```python
from build123d import *

# Parameters (mm, degrees)
F0_W     = 8
F0_H     = 3.175
F0_R     = 1.5
F0_W_2   = 3.175
F0_H_2   = 4
F0_R_2   = 1
F0_W_3   = 24
F0_H_3   = 12.5
F1_DEPTH = 3.175


# Not quite as in the source:
# - a length typed as a fraction of an inch, garbled in the dataset ("3 / 203.2 mm" for 3/8 in), is restored


with BuildPart() as f1:
    # F0 (on Top) → F1 (new body)
    with BuildSketch(Plane.XY):
        Polygon((-34.1063038088, 0.9337500209), (-34.1063038088, -28.6537499791), (9.0686961912, -28.6537499791), (9.0686961912, 0.9337500209), (-7.9313038088, 0.9337500209), (-7.9313038088, 20.1087500209), (-17.1063038088, 20.1087500209), (-17.1063038088, 0.9337500209), align=None)
        with Locations((-23.9313038088, -21.0662499791)):
            Rectangle(F0_W, F0_H, mode=Mode.SUBTRACT)
        with Locations((-29.5188038088, -10.9787499791)):
            Circle(F0_R, mode=Mode.SUBTRACT)
        with Locations((-29.5188038088, -4.4787499791)):
            Rectangle(F0_W_2, F0_H_2, mode=Mode.SUBTRACT)
        with Locations((-23.9313038088, -8.3162499791)):
            Circle(F0_R_2, mode=Mode.SUBTRACT)
        with Locations((-12.4313038088, -21.0662499791)):
            Circle(F0_R, mode=Mode.SUBTRACT)
        with Locations((-0.9313038088, -21.0662499791)):
            Rectangle(F0_W, F0_H, mode=Mode.SUBTRACT)
        with Locations((-9.4313038088, -8.3162499791)):
            Rectangle(F0_W_3, F0_H_3, mode=Mode.SUBTRACT)
        with Locations((5.0686961912, -8.3162499791)):
            Circle(F0_R_2, mode=Mode.SUBTRACT)
        with BuildLine():
            ThreePointArc((-14.1063038088, 15.5212500209), (-12.5188038088, 17.1087500209), (-10.9313038088, 15.5212500209))
            Line((-10.9313038088, 15.5212500209), (-10.9313038088, 2.5212500209))
            ThreePointArc((-10.9313038088, 2.5212500209), (-12.5188038088, 0.9337500209), (-14.1063038088, 2.5212500209))
            Line((-14.1063038088, 2.5212500209), (-14.1063038088, 15.5212500209))
        make_face(mode=Mode.SUBTRACT)
    extrude(amount=F1_DEPTH)


solid = f1.part
```
Geometry check sheet. Reference: the model listing, model coordinates, mm. A direction names the side the tool comes from. Coordinates: 2 decimals unless noted, no trailing zeros. Loops run counter-clockwise (first coordinate to the right, second up) from the corner with the lowest first, then second, coordinate; pieces in that order, holes last. Notation, with made-up numbers: (59, 83.25) - (109, 83.25) arc R15 ccw to (109, 104.25) - close; hole circle Ø2 at (83, 72.5). An arc over 180 degrees is marked (long way). One line per item, written item: value. Start each with the question number.
(1) Cross-section at B-B on y = -13.5. Enter the section's corners in (x, z) (3 decimals).
(2) Cross-section at C-C on x = -2.5. Enter the section's corners in (y, z) (3 decimals), plus the area to 3 significant figures.
(3) Depth check by flat-ended pin: P1, Ø1.6, axis at y = 12, z = 1, coming from the -X side; P2, Ø1.6, axis at y = 8, z = 1.5, coming from the +X side; P3, Ø1, axis at x = -3, z = 1.5, coming from the +Y side. Enter the tip coordinate at first touch or a pass-through.
(4) Cross-section at D-D on y = -20.5. Enter the section's corners in (x, z) (3 decimals), plus the area to 3 significant figures.
(5) Tool access check on faces 4 (the flat face through (-25, 0.934, 2)), 5 (the cylindrical face through (-12.55, 17.11, 1.57)), 6 (the flat face through (9.069, -14, 2)). Record the directions out of +Z, -Z, +X, -X, +Y, -Y that give a thin tool (end or side, any length) a straight path to the whole face; none if there is none.
(6) Mould release check, pull along Y, two halves, no side actions. Record for faces 1 (the flat face through (-13, -15, 3.175)), 2 (the flat face through (-27.931, -21, 2)), 3 (the flat face through (1, 0.934, 2)): released by +Y, released by -Y, zero draft, split by the parting line, or undercut.
(7) Material ranges on line 1 (Y direction, x = -21, z = 1.95); line 2 (Y direction, x = -10, z = 2.7); line 3 (Y direction, x = -26.5, z = 1.3), recorded low to high. Write a range as [from, to].
(8) Cross-section at A-A on x = -26. Enter the section's corners in (y, z) (3 decimals).
Results below:
1. outline: (-34.106, 0) - (-21.431, 0) - (-21.431, 3.175) - (-34.106, 3.175) - close; (2.569, 0) - (9.069, 0) - (9.069, 3.175) - (2.569, 3.175) - close
2. outline: (-28.654, 0) - (-22.654, 0) - (-22.654, 3.175) - (-28.654, 3.175) - close; (-19.479, 0) - (-14.566, 0) - (-14.566, 3.175) - (-19.479, 3.175) - close; (-2.066, 0) - (0.934, 0) - (0.934, 3.175) - (-2.066, 3.175) - close
2. area: 44.2 mm2
3. P1: stops at x = -17.11
3. P2: stops at x = -7.93
3. P3: stops at y = 0.93
4. outline: (-34.106, 0) - (-27.931, 0) - (-27.931, 3.175) - (-34.106, 3.175) - close; (-19.931, 0) - (-13.82, 0) - (-13.82, 3.175) - (-19.931, 3.175) - close; (-11.042, 0) - (-4.931, 0) - (-4.931, 3.175) - (-11.042, 3.175) - close; (3.069, 0) - (9.069, 0) - (9.069, 3.175) - (3.069, 3.175) - close
4. area: 77.5 mm2
5. face 4: +Z, -Z, -X, +Y
5. face 5: +Z, -Z
5. face 6: +Z, -Z, +X, +Y, -Y
6. face 1: zero draft
6. face 2: undercut
6. face 3: released by +Y
7. line 1: y = [-28.65, -22.65], [-19.48, -14.57], [-2.07, 0.93]
7. line 2: y = [-28.65, -14.57], [-2.07, 20.11]
7. line 3: y = [-28.65, -22.65], [-19.48, 0.93]
8. outline: (-28.654, 0) - (-22.654, 0) - (-22.654, 3.175) - (-28.654, 3.175) - close; (-19.479, 0) - (0.934, 0) - (0.934, 3.175) - (-19.479, 3.175) - close
